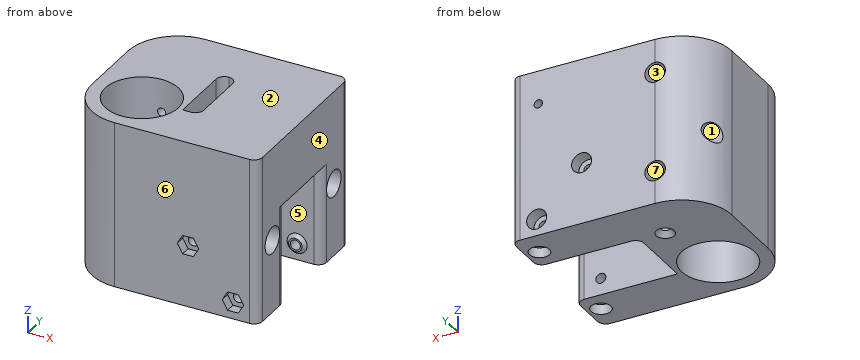
```python
from build123d import *

# Parameters (mm, degrees)
SKETCH1_W                = 58
SKETCH1_H                = 50
SKETCH1_R                = 11
BOSS_EXTRUDE1_DEPTH      = 50
SKETCH2_R                = 4
CUT_EXTRUDE1_DEPTH       = 20
SKETCH3_W                = 5
SKETCH3_H                = 21
CUT_EXTRUDE2_DEPTH       = 92.454906921
SKETCH14_W               = 25.5
SKETCH14_H               = 21
CUT_EXTRUDE9_DEPTH       = 30
SKETCH16_R               = 1.5
CUT_EXTRUDE10_DEPTH      = 57
CUT_EXTRUDE11_DEPTH      = 3
FILLET3_R                = 15
CUT_EXTRUDE12_REACH      = 93.455
SKETCH18_R               = 1.25
CUT_EXTRUDE13_REACH      = 93.455
CUT_EXTRUDE13_END_RADIUS = 11
SKETCH19_R               = 1.25
SKETCH20_R               = 3
CUT_EXTRUDE14_DEPTH      = 10
SKETCH21_R               = 3
CUT_EXTRUDE15_DEPTH      = 3
FILLET4_R                = 2.5
SKETCH22_R               = 1.25
CUT_EXTRUDE16_DEPTH      = 81.274529133
SKETCH23_R               = 3
CUT_EXTRUDE17_DEPTH      = 10
SKETCH24_R               = 3
CUT_EXTRUDE18_DEPTH      = 4
SKETCH25_R               = 1.25
CUT_EXTRUDE19_DEPTH      = 10
SKETCH26_R               = 3
SKETCH26_R_2             = 1.5
BOSS_EXTRUDE2_DEPTH      = 1
BOSS_EXTRUDE3_START      = 1
SKETCH27_R               = 3
SKETCH27_R_2             = 1.5
BOSS_EXTRUDE3_DEPTH      = 1
CHAMFER1_SIZE            = 1
SKETCH28_R               = 1.25
CUT_EXTRUDE20_DEPTH      = 10
CHAMFER2_SIZE            = 1.5


with BuildPart() as part:
    # Sketch1 → Boss-Extrude1 (new body)
    with BuildSketch(Plane.XY):
        with Locations((29, 25)):
            Rectangle(SKETCH1_W, SKETCH1_H)
        with Locations((15, 15)):
            Circle(SKETCH1_R, mode=Mode.SUBTRACT)
    extrude(amount=BOSS_EXTRUDE1_DEPTH)

    # Sketch2 → Cut-Extrude1 (cut)
    with BuildSketch(Plane.ZY.offset(-58)):
        with Locations((22, 42)):
            Circle(SKETCH2_R)
        with Locations((22, 8)):
            Circle(SKETCH2_R)
    extrude(amount=CUT_EXTRUDE1_DEPTH, mode=Mode.SUBTRACT)

    # Sketch3 → Cut-Extrude2 (cut, through all)
    with BuildSketch(Plane(origin=(0, 0, 0), x_dir=(-1, 0, 0), z_dir=(0, 0, -1))):
        with Locations((-30, 25)):
            Rectangle(SKETCH3_W, SKETCH3_H)
    extrude(amount=-CUT_EXTRUDE2_DEPTH, mode=Mode.SUBTRACT)

    # Sketch14 → Cut-Extrude9 (cut)
    with BuildSketch(Plane(origin=(0, 0, 0), x_dir=(-1, 0, 0), z_dir=(0, 0, -1))):
        with Locations((-45.25, 25)):
            Rectangle(SKETCH14_W, SKETCH14_H)
    extrude(amount=-CUT_EXTRUDE9_DEPTH, mode=Mode.SUBTRACT)

    # Sketch16 → Cut-Extrude10 (cut)
    with BuildSketch(Plane(origin=(0, 50, 0), x_dir=(1, 0, 0), z_dir=(0, 1, 0))):
        with Locations(Location((50.5, -5, 0), (0, 0, 270))):
            Circle(SKETCH16_R)
        with Locations(Location((37, -18.5, 0), (0, 0, 270))):
            Circle(SKETCH16_R)
    extrude(amount=-CUT_EXTRUDE10_DEPTH, mode=Mode.SUBTRACT)

    # Sketch17 → Cut-Extrude11 (cut)
    with BuildSketch(Plane.XZ):
        Polygon((38.616580754, 15.7), (40.233161507, 18.5), (38.616580754, 21.3), (35.383419246, 21.3), (33.766838493, 18.5), (35.383419246, 15.7), align=None)
        Polygon((53.733161507, 5), (52.116580754, 7.8), (48.883419246, 7.8), (47.266838493, 5), (48.883419246, 2.2), (52.116580754, 2.2), align=None)
    extrude(amount=-CUT_EXTRUDE11_DEPTH, mode=Mode.SUBTRACT)

    # Fillet3
    fillet3_edges = [part.edges().sort_by_distance(p)[0] for p in [
        (0, 50, 25),
        (0, 0, 25),
    ]]
    fillet(fillet3_edges, radius=FILLET3_R)

    # Sketch18 → Cut-Extrude12 (cut, up to next)
    with BuildSketch(Plane(origin=(0, 0, 0), x_dir=(-1, 0, 0), z_dir=(0, 0, -1)), mode=Mode.PRIVATE) as cut_extrude12_sk1:
        with Locations((-54, 42)):
            Circle(SKETCH18_R)
    cut_extrude12_tool1 = extrude(cut_extrude12_sk1.sketch, amount=-CUT_EXTRUDE12_REACH, mode=Mode.PRIVATE) & part.part
    # Sketch18 → Cut-Extrude12 (cut, up to next)
    with BuildSketch(Plane(origin=(0, 0, 0), x_dir=(-1, 0, 0), z_dir=(0, 0, -1)), mode=Mode.PRIVATE) as cut_extrude12_sk2:
        with Locations((-54, 8)):
            Circle(SKETCH18_R)
    cut_extrude12_tool2 = extrude(cut_extrude12_sk2.sketch, amount=-CUT_EXTRUDE12_REACH, mode=Mode.PRIVATE) & part.part
    add(cut_extrude12_tool1.solids().sort_by_distance((54, 42, 0))[0], mode=Mode.SUBTRACT)
    add(cut_extrude12_tool2.solids().sort_by_distance((54, 8, 0))[0], mode=Mode.SUBTRACT)

    # Cut-Extrude13: up to this cylinder (the profile starts outside it)
    cut_extrude13_end = Plane(origin=(15, 15, 25), z_dir=(0, 0, -1)) * Cylinder(CUT_EXTRUDE13_END_RADIUS, 239.91, mode=Mode.PRIVATE)
    # Sketch19 → Cut-Extrude13 (cut, up to the surface)
    with BuildSketch(Plane(origin=(0, 50, 0), x_dir=(1, 0, 0), z_dir=(0, 1, 0)), mode=Mode.PRIVATE) as cut_extrude13_sk1:
        with Locations(Location((15, -10, 0), (0, 0, 270))):
            Circle(SKETCH19_R)
    cut_extrude13_tool1 = extrude(cut_extrude13_sk1.sketch, amount=-CUT_EXTRUDE13_REACH, mode=Mode.PRIVATE) - cut_extrude13_end
    add(cut_extrude13_tool1.solids().sort_by_distance((15, 50, 10))[0], mode=Mode.SUBTRACT)
    # Sketch19 → Cut-Extrude13 (cut, up to the surface)
    with BuildSketch(Plane(origin=(0, 50, 0), x_dir=(1, 0, 0), z_dir=(0, 1, 0)), mode=Mode.PRIVATE) as cut_extrude13_sk2:
        with Locations(Location((15, -40, 0), (0, 0, 270))):
            Circle(SKETCH19_R)
    cut_extrude13_tool2 = extrude(cut_extrude13_sk2.sketch, amount=-CUT_EXTRUDE13_REACH, mode=Mode.PRIVATE) - cut_extrude13_end
    add(cut_extrude13_tool2.solids().sort_by_distance((15, 50, 40))[0], mode=Mode.SUBTRACT)

    # Sketch20 → Cut-Extrude14 (cut)
    with BuildSketch(Plane(origin=(0, 50, 0), x_dir=(1, 0, 0), z_dir=(0, 1, 0))):
        with Locations(Location((15, -10, 0), (0, 0, 270))):
            Circle(SKETCH20_R)
        with Locations(Location((15, -40, 0), (0, 0, 270))):
            Circle(SKETCH20_R)
    extrude(amount=-CUT_EXTRUDE14_DEPTH, mode=Mode.SUBTRACT)

    # Sketch21 → Cut-Extrude15 (cut)
    with BuildSketch(Plane(origin=(0, 0, 0), x_dir=(-1, 0, 0), z_dir=(0, 0, -1))):
        with Locations((-54, 42)):
            Circle(SKETCH21_R)
        with Locations((-54, 8)):
            Circle(SKETCH21_R)
    extrude(amount=-CUT_EXTRUDE15_DEPTH, mode=Mode.SUBTRACT)

    # Fillet4
    fillet4_edges = [part.edges().sort_by_distance(p)[0] for p in [
        (32.5, 35.5, 40),
        (32.5, 14.5, 40),
        (58, 0, 25),
        (58, 14.5, 15),
        (27.5, 35.5, 25),
        (58, 35.5, 15),
        (58, 50, 25),
    ]]
    fillet(fillet4_edges, radius=FILLET4_R - 0.0001)  # a hair under: the kernel refuses the full size

    # Sketch22 → Cut-Extrude16 (cut, through all)
    with BuildSketch(Plane(origin=(38, 0, 0), x_dir=(0, 0, -1), z_dir=(1, 0, 0))):
        with Locations((-22, 42)):
            Circle(SKETCH22_R)
    extrude(amount=-CUT_EXTRUDE16_DEPTH, mode=Mode.SUBTRACT)

    # Sketch23 → Cut-Extrude17 (cut)
    with BuildSketch(Plane.ZY):
        with Locations((22, 42)):
            Circle(SKETCH23_R)
    extrude(amount=-CUT_EXTRUDE17_DEPTH, mode=Mode.SUBTRACT)

    # Sketch24 → Cut-Extrude18 (cut)
    with BuildSketch(Plane(origin=(0, 50, 0), x_dir=(1, 0, 0), z_dir=(0, 1, 0))):
        with Locations(Location((50.5, -5, 0), (0, 0, 270))):
            Circle(SKETCH24_R)
        with Locations(Location((37, -18.5, 0), (0, 0, 270))):
            Circle(SKETCH24_R)
    extrude(amount=-CUT_EXTRUDE18_DEPTH, mode=Mode.SUBTRACT)

    # Sketch25 → Cut-Extrude19 (cut)
    with BuildSketch(Plane(origin=(0, 50, 0), x_dir=(1, 0, 0), z_dir=(0, 1, 0))):
        with Locations(Location((50, -40, 0), (0, 0, 270))):
            Circle(SKETCH25_R)
    extrude(amount=-CUT_EXTRUDE19_DEPTH, mode=Mode.SUBTRACT)

    # Sketch26 → Boss-Extrude2 (add)
    with BuildSketch(Plane.XZ.offset(-35.5)):
        with Locations(Location((50.5, 5, 0), (0, 0, 90))):
            Circle(SKETCH26_R)
        with Locations(Location((50.5, 5, 0), (0, 0, 90))):
            Circle(SKETCH26_R_2, mode=Mode.SUBTRACT)
    extrude(amount=BOSS_EXTRUDE2_DEPTH)

    # Sketch27 → Boss-Extrude3 (add)
    with BuildSketch(Plane(origin=(0, 14.5, 0), x_dir=(1, 0, 0), z_dir=(0, 1, 0)).offset(BOSS_EXTRUDE3_START)):
        with Locations(Location((37, -18.5, 0), (0, 0, 270))):
            Circle(SKETCH27_R)
        with Locations(Location((37, -18.5, 0), (0, 0, 270))):
            Circle(SKETCH27_R_2, mode=Mode.SUBTRACT)
    extrude(amount=-BOSS_EXTRUDE3_DEPTH)

    # Chamfer1
    chamfer1_edges = [part.edges().sort_by_distance(p)[0] for p in [
        (50.5, 34.5, 2),
        (37, 15.5, 15.5),
    ]]
    chamfer(chamfer1_edges, length=CHAMFER1_SIZE - 0.0001)  # a hair under: the kernel refuses the full size

    # Sketch28 → Cut-Extrude20 (cut)
    with BuildSketch(Plane(origin=(0, 0, 0), x_dir=(-1, 0, 0), z_dir=(0, 0, -1))):
        with Locations((-20.088889062, 34.9)):
            Circle(SKETCH28_R)
    extrude(amount=-CUT_EXTRUDE20_DEPTH, mode=Mode.SUBTRACT)

    # Chamfer2
    chamfer2_edges = [part.edges().sort_by_distance(p)[0] for p in [
        (21.338889062, 34.9, 0),
    ]]
    chamfer(chamfer2_edges, length=CHAMFER2_SIZE)


solid = part.part
```
Check sheet for the modelled part. Datum: model origin and axes. Units: mm. Face numbers are marked on the shaded views. A direction names the side the tool comes from. Coordinates: 2 decimals unless noted, no trailing zeros. Order: outer loops, then holes, each group sorted by start corner. A loop starts at its lowest first (then second) coordinate and runs counter-clockwise, first axis right, second up. Notation, with made-up numbers: M 28.5,33.25 L 85.5,33.25 A18 ccw 85.5,64.25 Z; hole C -35,16 d6. An arc over 180 degrees is marked long. Write each question's results on one line, items separated by ' | '. Start each with the question number.
1. Cross-section at A-A on x = 37. State how many separate pieces and enclosed holes the cut face has, and give its area (3 significant figures).
2. Cross-section at C-C on x = 11. Record the cut outline in (y, z), and give its area (3 significant figures).
3. Mould release check, pull along Z, two halves, no side actions. Record for the marked faces 1, 2, 3 and 4: +Z half, -Z half, draft (parallel to the pull), parting line (faces both ways), or undercut.
4. Material ranges on probe 1 along Y at (x, z) = (33, 29.5); probe 2 along X at (y, z) = (28, 10); probe 3 along X at (y, z) = (30, 30.5), recorded low to high.
5. Go/stop test with flat-tipped pins: P1, Ø1.2, axis at x = 50, z = 39.5, coming from the +Y side; P2, Ø3, axis at x = 20.09, y = 34.9, coming from the -Z side; P3, Ø5, axis at x = 6.5, z = 40, coming from the -Y side. Record where each tip stops, or that it passes through.
6. Cross-section at B-B on y = 30. Record the cut outline in (x, z).
7. Access from +Z, -Z, +X, -X, +Y, -Y to the whole of each face (thin tool, end or side, straight path). Record for the marked faces 5, 6 and 7.
8. Cross-section at D-D on y = 8. Record the cut outline in (x, z).
Checks:
1) separate pieces: 3 | enclosed holes: 1 | area: 1,760 mm²
2) outline: M 0.54,0 L 4.75,0 L 4.75,50 L 0.54,50 Z; M 25.25,0 L 49.46,0 L 49.46,50 L 25.25,50 Z; hole C 42,22 d2.5 | area: 1,420 mm²
3) face 1: undercut | face 2: +Z half | face 3: undercut | face 4: draft
4) probe 1: y = 0 to 14.5, 35.5 to 50 | probe 2: x = 0 to 13.75, 16.25 to 27.5 | probe 3: x = 0 to 27.5, 32.5 to 58
5) P1: stops at y = 40 | P2: stops at z = 1.25 | P3: stops at y = 1.25
6) outline: M 0,0 L 27.5,0 L 27.5,50 L 0,50 Z; M 32.5,30 L 58,30 L 58,50 L 32.5,50 Z; hole C 15,10 d2.5; hole C 15,40 d2.5
7) face 5: none | face 6: +Z, -Z, +X, -X, -Y | face 7: +Y
8) outline: M 1.73,0 L 6.51,0 L 6.51,50 L 1.73,50 Z; M 23.49,0 L 51,0 L 51,3 L 52.75,3 L 52.75,18 L 38.41,18 A1.5 cw long 38,19.62 L 38,26 L 58,26 L 58,50 L 23.49,50 Z; M 55.25,3 L 57,3 L 57,0 L 58,0 L 58,18 L 55.25,18 Z; hole C 50.5,5 d3
